The listing builds one solid part. Answer for the finished solid, in the listing's coordinates (mm). A direction names the side the tool comes from. Round coordinates to 2 decimals unless told otherwise and drop trailing zeros. Write each loop counter-clockwise with the first axis right and the second up, starting at its lowest first coordinate (ties: lowest second). Pieces come first, ordered by that corner, then holes. Notation, with made-up numbers: (4.25, 3.25) - (45.25, 3.25) arc R6 ccw to (45.25, 7.25) - close; hole circle Ø3 at (87, -26). An arc over 180 degrees is marked (long way). Use a Markdown table: item, result. Add a question column.
1) A cutting plane is placed at A-A (z = 22.5). Give the vertices of the cut face in (x, y) (3 decimals), then the cut area to 3 significant figures.
2) A cutting plane is placed at D-D (x = 7.5). Give the vertices of the cut face in (y, z).
3) A cutting plane is placed at C-C (x = -10). Give the vertices of the cut face in (y, z), then the cut area to 3 significant figures.
4) Each of these flat-tipped pins is pushed along its axis until it touches: P1, Ø5, axis at y = 7, z = 8.5, coming from the -X side; P2, Ø5, axis at x = -5, y = 5, coming from the -Z side; P3, Ø5, axis at x = -12, y = 4.5, coming from the +Z side. Where does it stop, or does it pass through?
5) A cutting plane is placed at B-B (y = 5). State how many separate pieces and enclosed holes the cut face has, then the cut area to 3 significant figures.
6) Find the intervals of material crossed by probe 1 along X at (y, z) = (6.75, 62); probe 2 along Y at (x, z) = (-36.4, 18) (3 decimals); probe 3 along Z at (x, y) = (-39, 3), in increasing order. Write a range as from..to.
7) Determine the mould class of faces 3 (the flat face through (7, 5, 0)), 4 (the cylindrical face through (7.175, 5.07, 63.664)), 5 (the flat face through (1, 0, 43)), 6 (the flat face through (-21, 5, 30)) for opening direction Z: +Z half, -Z half, draft (parallel to the pull), parting line (faces both ways), or undercut.
8) A tool of negligible diameter and unlimited length cuts with its end or side. For faces 1 (the flat face through (0, 5, 71)), 2 (the cylindrical face through (6.3, 5.1, 7.4)), from which of +Z, -Z, +X, -X, +Y, -Y can it reach the whole face along a straight path? Write none if from no direction.
Autodesk Inventor part; units mm, degrees
ref_plane "YZ Plane" through (0, 0, 0) normal (1, 0, 0) x (0, 1, 0)
ref_plane "XZ Plane" through (0, 0, 0) normal (0, 1, 0) x (-1, 0, 0)
ref_plane "XY Plane" through (0, 0, 0) normal (0, 0, 1) x (1, 0, 0)
sketch "Sketch1" plane through (0, 0, 0) normal (0, 0, 1) x (1, 0, 0)
  line L0 (0, 0) -> (15, 0)
  line L1 (15, 0) -> (15, 10)
  line L2 (15, 10) -> (0, 10)
  line L3 (0, 10) -> (0, 0)
  line L4 (1, 9) -> (14, 9)
  line L5 (14, 9) -> (14, 1)
  line L6 (14, 1) -> (1, 1)
  line L7 (1, 1) -> (1, 9)
  dimension "d0" = 15
  dimension "d1" = 10
  dimension "d2" = 13
  dimension "d3" = 8
  dimension "d4" = 1
  dimension "d5" = 1
extrude "Extrusion1" add sketch "Sketch1" along normal blind 112.5 contours L3 L2 L1 L0 | L4 L5 L6 L7
sketch "Sketch2" plane through (0, 10, 0) normal (0, 1, 0) x (1, 0, 0)
  line L0 (15, 0) -> (0, 0)
  line L1 (0, 0) -> (0, -112.5)
  line L2 (15, -112.5) -> (0, -112.5)
  line L3 (15, 0) -> (15, -112.5)
  circle A0 centre (7.5, -6.5) radius 1.5
  circle A1 centre (7.5, -98.2) radius 1.5
  circle A2 centre (7.5, -19.5) radius 1.5
  circle A3 centre (7.5, -88.2) radius 1.5
  circle A4 centre (7.5, -78.2) radius 1.5
  circle A5 centre (7.5, -62.2) radius 1.5
  dimension "d8" = 3
  dimension "d9" = 3
  dimension "d10" = 7.5
  dimension "d11" = 7.5
  dimension "d13" = 14.3
  dimension "d24" = 3
  dimension "d25" = 3
  dimension "d26" = 3
  dimension "d27" = 3
  dimension "d28" = 7.5
  dimension "d29" = 7.5
  dimension "d30" = 7.5
  dimension "d31" = 7.5
  dimension "d32" = 13
  dimension "d33" = 10
  dimension "d34" = 10
  dimension "d35" = 16
  dimension "d55" = 6.5
extrude "Extrusion2" cut sketch "Sketch2" against normal up to surface (10 mm away) contours A0 | A1 | A2 | A3 | A4 | A5
sketch "Sketch3" plane through (15, 0, 0) normal (1, 0, 0) x (0, 0, -1)
  line L0 (0, 0) -> (0, 10)
  line L1 (0, 10) -> (-112.5, 10)
  line L2 (-112.5, 0) -> (-112.5, 10)
  line L3 (0, 0) -> (-112.5, 0)
  circle A0 centre (-9, 5) radius 1.5
  circle A1 centre (-107.5, 5) radius 1.5
  dimension "d16" = 3
  dimension "d17" = 5
  dimension "d18" = 9
  dimension "d21" = 3
  dimension "d22" = 5
  dimension "d23" = 5
extrude "Extrusion3" [suppressed]
sketch "Sketch4" plane through (0, 10, 0) normal (0, 1, 0) x (1, 0, 0)
  circle A0 centre (7.5, -62.2) radius 1.5
  circle A1 centre (7.5, -88.2) radius 1.5
  circle A2 centre (7.5, -98.2) radius 1.5
  circle A3 centre (7.5, -19.5) radius 1.5
  circle A4 centre (7.5, -78.2) radius 1.5
  circle A5 centre (7.5, -6.5) radius 1.5
  line L0 (15, 0) -> (0, 0)
  line L1 (0, 0) -> (0, -112.5)
  line L2 (15, -112.5) -> (0, -112.5)
  line L3 (15, 0) -> (15, -112.5)
  line L4 (0, 0) -> (0, -112.5)
  line L5 (0, -15) -> (-41.4, -15)
  line L6 (-41.4, -15) -> (-41.4, -30)
  line L7 (-41.4, -30) -> (0, -30)
  line L8 (0, -30) -> (0, -15)
  circle A6 centre (-10, -22.5) radius 1.5
  circle A7 centre (-31.4, -22.5) radius 1.5
  point P0 (0, -30)
  dimension "d36" = 15
  dimension "d37" = 15
  dimension "d38" = 41.4
  dimension "d39" = 3
  dimension "d40" = 3
  dimension "d41" = 7.5
  dimension "d42" = 7.5
  dimension "d43" = 10
  dimension "d44" = 10
extrude "Extrusion4" add sketch "Sketch4" against normal blind 10 contours L1 L7 L6 L5
sketch "Sketch5" plane through (-41.4, 10, 30) normal (0, 0, 1) x (1, 0, 0)
  line L0 (0, 0) -> (41.4, 0)
  line L1 (0, 0) -> (0, -10)
  line L2 (41.4, -10) -> (0, -10)
  line L3 (41.4, 0) -> (41.4, -10)
  circle A0 centre (5, -5) radius 1.625
  circle A1 centre (36.4, -5) radius 1.625
  point P0 (41.4, -10)
  dimension "d47" = 3.25
  dimension "d48" = 3.25
  dimension "d49" = 5
  dimension "d50" = 5
  dimension "d51" = 5
  dimension "d52" = 5
extrude "Extrusion5" cut sketch "Sketch5" against normal up to surface (15 mm away) contours A0 | A1
properties part number "profile4_3D" material "Aluminum 6061, Welded"
Entries:
| question | item | result |
|---|---|---|
| 1 | outline | (-41.4, 0) - (-32.9, 0) - (-32.9, 10) - (-41.4, 10) - close; (-29.9, 0) - (-11.5, 0) - (-11.5, 10) - (-29.9, 10) - close; (-8.5, 0) - (15, 0) - (15, 10) - (-8.5, 10) - close; hole circle Ø3.25 at (-36.4, 5); hole circle Ø3.25 at (-5, 5) |
| 1 | area | 487 mm² |
| 2 | outline | (0, 0) - (10, 0) - (10, 5) - (0, 5) - close; (0, 8) - (10, 8) - (10, 18) - (0, 18) - close; (0, 21) - (10, 21) - (10, 60.7) - (0, 60.7) - close; (0, 63.7) - (10, 63.7) - (10, 76.7) - (0, 76.7) - close; (0, 79.7) - (10, 79.7) - (10, 86.7) - (0, 86.7) - close; (0, 89.7) - (10, 89.7) - (10, 96.7) - (0, 96.7) - close; (0, 99.7) - (10, 99.7) - (10, 112.5) - (0, 112.5) - close |
| 3 | outline | (0, 15) - (10, 15) - (10, 21) - (0, 21) - close; (0, 24) - (10, 24) - (10, 30) - (0, 30) - close |
| 3 | area | 120 mm² |
| 4 | P1 | stops at x = 0 |
| 4 | P2 | stops at z = 15 |
| 4 | P3 | stops at z = 30 |
| 5 | separate pieces | 3 |
| 5 | enclosed holes | 8 |
| 5 | area | 2,150 mm² |
| 6 | probe 1 | x = 0..6.01, 8.99..15 |
| 6 | probe 2 | y = 0..3.375, 6.625..10 |
| 6 | probe 3 | z = 15..30 |
| 7 | face 3 | -Z half |
| 7 | face 4 | undercut |
| 7 | face 5 | draft |
| 7 | face 6 | +Z half |
| 8 | face 1 | +Z, -X, +Y, -Y |
| 8 | face 2 | +Y, -Y |
